```python
from build123d import *

# Parameters (mm, degrees)
F3_ANGLE = 180
F8_DEPTH = 869.6470786003
F9_T     = -6.35


with BuildPart() as f2:
    # F0 (on Front) → F2 section 0
    with BuildSketch(Plane.XZ, mode=Mode.PRIVATE) as f2_s0:
        Polygon((0, -1479.5302793129), (1407.1169131965, -457.2), (869.6460785003, 1196.9651396565), (-869.6460785003, 1196.9651396565), (-1258.5636280788, 0), (-1407.1169131965, -457.2), align=None)
    loft([f2_s0.sketch, Vertex(0, -2393.9302793129, 0)])


with BuildPart() as f3_1:
    # F3: copy of F2
    add(f2.part.rotate(Axis((98.339766264, -739.7651396565, 0), (1, 0, 0)), F3_ANGLE))


with BuildPart() as f2_1:
    add(f2.part)

    # F4: intersect F3_1
    add(f3_1.part, mode=Mode.INTERSECT)

    # F7 (on 3pt) → F8 (cut, through all)
    with BuildSketch(Plane(origin=(0, 0, 0), x_dir=(0, -1, 0), z_dir=(-1, 0, 0))):
        Polygon((1784.3302793129, 645.576759771), (549.4445933651, 1263.0196027449), (-304.8, 735.0674093394), (-304.8, -441.1666341224), (904.9484231668, -1278.5552855277), (1784.3302793129, -735.0674093394), align=None)
        Polygon((0, 565.1302793129), (565.1302793129, 914.4), (1479.5302793129, 457.2), (1479.5302793129, -565.1302793129), (914.4, -914.4), (0, -281.4517206871), align=None, mode=Mode.SUBTRACT)
        Polygon((1479.5302793129, 457.2), (565.1302793129, 914.4), (0, 565.1302793129), (0, -281.4517206871), (914.4, -914.4), (1479.5302793129, -565.1302793129), align=None)
    extrude(amount=F8_DEPTH, mode=Mode.SUBTRACT)

    # F9
    f9_openings = [f2_1.faces().sort_by_distance(p)[0] for p in [
        (0, -739.76514, 0),
    ]]
    offset(amount=F9_T, openings=f9_openings)


solid = f2_1.part
```
Input: part model. Units: mm. Frame: model coordinates. A direction names the side the tool comes from. Round coordinates to 2 decimals unless told otherwise and drop trailing zeros. Loops run counter-clockwise (first coordinate to the right, second up) from the corner with the lowest first, then second, coordinate; pieces in that order, holes last. Notation, with made-up numbers: (43.5, -20.75) -> (81.5, -20.75) arc R24 cw to (81.5, 8.25) -> close; hole circle Ø3 at (-7, -36.75). An arc over 180 degrees is marked (long way). One line per item, written item: value.
(1) Pin query (flat end, axial travel): pin 1 (1 mm diameter, centred on x = 111, y = -635.5, fed in from +Z); pin 2 (1.5 mm diameter, centred on y = -1104.5, z = 413.5, fed in from +X); pin 3 (1.5 mm diameter, centred on y = -784, z = -436.5, fed in from -X). Return the tip coordinate at first contact, or that it passes through.
Geometry check:
pin 1: z = 877.72
pin 2: x = 544
pin 3: x = 743.15
(2) Set-up query: faces 1 (the face through (645.924, -1026.251, 202.029)), 2 (the face through (395.13, -450.8, 556.66)). Return all of +Z, -Z, +X, -X, +Y, -Y with unobstructed straight access to the full face (end or side cutting, diameter ignored); none if empty.
Geometry check:
face 1: -X
face 2: +Z, +X, +Y
(3) Section D-D (z = -690.5). Return the cut outline in (x, y), plus the area to 3 significant figures.
Geometry check:
outline: (0, -1276.68) -> (573.26, -602.77) -> (501.68, -466.6) -> (0, -466.6) -> (0, -480.8) -> (501.68, -480.8) -> (564.04, -599.41) -> (0, -1262.48) -> close
area: 16,100 mm2
(4) Material intervals for line 1 (Y direction, x = 98.5, z = 24.5); line 2 (Y direction, x = 441, z = -556); line 3 (Z direction, x = 301, y = -485), sorted ascending. Write a range as [from, to].
Geometry check:
line 1: [-1479.53, -1473.18], [-6.35, 0]
line 2: [-975.88, -961.68], [-282.26, -268.06]
line 3: [-699.7, -692.6], [637.41, 646.19]
(5) Section A-A (x = 442). Return the cut outline in (y, z).
Geometry check:
outline: (-1479.53, -244) -> (-627.17, -770.79) -> (-302.32, -608.36) -> (0, -119.19) -> (0, 244) -> (-852.36, 770.79) -> (-1177.21, 608.36) -> (-1479.53, 119.19) -> close; hole (-1473.18, -239.15) -> (-625.67, -762.94) -> (-316.52, -608.36) -> (-6.35, -106.49) -> (-6.35, 239.15) -> (-853.86, 762.94) -> (-1163.01, 608.36) -> (-1473.18, 106.49) -> close
(6) Mould query, pull axis Y, two halves, no side actions, for faces 3 (the face through (395.1, -1028.7, -556.7)), 4 (the face through (651.516, -450.799, -203.779)), 5 (the face through (391.74, -453.28, 551.88)). Classes: pulls with the +Y half, pulls with the -Y half, needs draft (parallel to the pull), parting line crosses it, or undercut.
Geometry check:
face 3: pulls with the -Y half
face 4: pulls with the +Y half
face 5: undercut
(7) Section B-B (z = 308.5). Return the cut outline in (x, y).
Geometry check:
outline: (0, -1479.53) -> (380.49, -1479.53) -> (850.8, -584.94) -> (353.22, 0) -> (0, 0) -> (0, -6.35) -> (346.54, -6.35) -> (841.58, -588.29) -> (376.36, -1473.18) -> (0, -1473.18) -> close
(8) Section C-C (y = -959.5). Return the cut outline in (x, z), plus the area to 3 significant figures.
Geometry check:
outline: (0, -886.53) -> (843.14, -273.95) -> (521.09, 717.22) -> (0, 717.22) -> (0, 710.12) -> (515.93, 710.12) -> (834.79, -271.24) -> (0, -877.75) -> close
area: 18,400 mm2
